Here's how the part is built. I have some questions about the finished solid (model axes, mm). Coordinates: 2 decimals unless noted, no trailing zeros. Write each loop counter-clockwise with the first axis right and the second up, starting at its lowest first coordinate (ties: lowest second). Pieces come first, ordered by that corner, then holes. Notation, with made-up numbers: (41, 83.5) -> (64, 83.5) arc R34 cw to (64, 122.5) -> close; hole circle Ø11 at (43, 31). An arc over 180 degrees is marked (long way). Put each result on its own line as item: value. Start each with the question number.
Item 1: I need wall thicknesses on line 1 (Z direction, x = 81.5, y = 6.5); line 2 (X direction, y = 9, z = -7); line 3 (Z direction, x = 82, y = 8.5). Which ranges of each line are inside material? Lowest first, please. Write a range as [from, to].
Item 2: I want a section at A-A, the plane y = 3. List the corners of the cut face in (x, z) for me, then the cut area to 3 significant figures.
Item 3: For pin 1 (3 mm diameter, centred on x = 31, y = 8.5, fed in from -Z); pin 2 (3 mm diameter, centred on x = -59, y = 8, fed in from +Z), each with a flat end and sliding along its axis, tell me the tip position at first contact or that it passes through.
from build123d import *

# Parameters (mm, degrees)
DODANIE_WYCI_GNI_CIE1_DEPTH = 10
ZAOKR_GLENIE1_R             = 4


with BuildPart() as part:
    # Szkic1 → Dodanie-wyciągnięcie1 (new body)
    with BuildSketch(Plane(origin=(0, 0, 0), x_dir=(1, 0, 0), z_dir=(0, 1, 0))):
        with BuildLine():
            Line((-110, -100), (110, -100))
            ThreePointArc((110, -100), (138.284271247, -88.284271247), (150, -60))
            Line((150, -60), (150, 60))
            ThreePointArc((150, 60), (138.284271247, 88.284271247), (110, 100))
            Line((110, 100), (-110, 100))
            ThreePointArc((-110, 100), (-138.284271247, 88.284271247), (-150, 60))
            Line((-150, 60), (-150, -60))
            ThreePointArc((-150, -60), (-138.284271247, -88.284271247), (-110, -100))
        make_face()
    extrude(amount=DODANIE_WYCI_GNI_CIE1_DEPTH)

    # Zaokrąglenie1
    zaokr_glenie1_edges = [part.edges().sort_by_distance(p)[0] for p in [
        (-138.284271247, 10, -88.284271247),
        (-150, 10, 0),
        (-138.284271247, 10, 88.284271247),
        (0, 10, 100),
        (138.284271247, 10, 88.284271247),
        (150, 10, 0),
        (138.284271247, 10, -88.284271247),
        (0, 10, -100),
    ]]
    fillet(zaokr_glenie1_edges, radius=ZAOKR_GLENIE1_R)


solid = part.part
Calculated:
1. line 1: z = [-99.97, 99.97]
1. line 2: x = [-148.65, 148.65]
1. line 3: z = [-99.12, 99.12]
2. outline: (-150, -60) arc R40 ccw to (-110, -100) -> (110, -100) arc R40 ccw to (150, -60) -> (150, 60) arc R40 ccw to (110, 100) -> (-110, 100) arc R40 ccw to (-150, 60) -> close
2. area: 58,600 mm2
3. pin 1: stops at z = -99.87
3. pin 2: stops at z = 99.97
